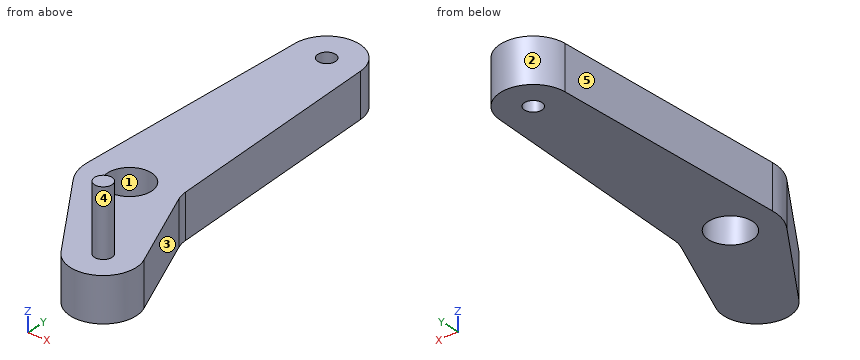
```python
from build123d import *

# Parameters (mm, degrees)
SKETCH_1_R      = 10
SKETCH_1_R_2    = 4
EXTRUDE_1_DEPTH = 20
SKETCH_2_R      = 4
EXTRUDE_2_DEPTH = 30


with BuildPart() as part:
    # 草图1 → 凸台-拉伸1 (new body)
    with BuildSketch(Plane.XY):
        with BuildLine():
            Line((-14.98449612, 110.681818182), (-19.97932816, 0.909090909))
            ThreePointArc((-19.97932816, 0.909090909), (-19.236072743, -5.474806428), (-16.506376679, -11.293340025))
            Line((-16.506376679, -11.293340025), (11.58545194, -52.352433595))
            ThreePointArc((11.58545194, -52.352433595), (31.154804784, -57.04715715), (37.782931026, -38.045369273))
            Line((37.782931026, -38.045369273), (20.861374384, 2.011947794))
            ThreePointArc((20.861374384, 2.011947794), (20.049111843, 4.537769231), (19.694574841, 7.167188916))
            Line((19.694574841, 7.167188916), (14.98449612, 110.681818182))
            ThreePointArc((14.98449612, 110.681818182), (0, 125), (-14.98449612, 110.681818182))
        make_face()
        Circle(SKETCH_1_R, mode=Mode.SUBTRACT)
        with Locations((0, 110)):
            Circle(SKETCH_1_R_2, mode=Mode.SUBTRACT)
    extrude(amount=EXTRUDE_1_DEPTH)

    # 草图2 → 凸台-拉伸2 (add)
    with BuildSketch(Plane.XY.offset(20)):
        with Locations((23.965234449, -43.882428577)):
            Circle(SKETCH_2_R)
    extrude(amount=EXTRUDE_2_DEPTH)


solid = part.part
```
Input: part model. Units: mm. Frame: model coordinates. Face numbers are marked on the shaded views. A direction names the side the tool comes from. Give positions to 0.01 mm unless a question says otherwise; leave off trailing zeros. Loops run counter-clockwise (first coordinate to the right, second up) from the corner with the lowest first, then second, coordinate; pieces in that order, holes last. Notation, with made-up numbers: M 24,-10.5 L 35,-10.5 A30 cw 35,16.5 Z; hole C -33,19.5 d6. An arc over 180 degrees is marked long. Answer as CSV lines item,"result". Start each with the question number.
1. Section B-B on z = 12. Return loops of the section in (x, y).
2. Line query: L1, parallel to Y at x = 24, z = 27; L2, parallel to Z at x = 2, y = -36; L3, parallel to Y at x = 33.5, z = 5. Output: solid intervals per line, ascending.
3. Pin query (flat end, axial travel): P1, Ø1.5, axis at y = 12.5, z = 17, coming from the -X side; P2, Ø10, axis at x = -2, z = 20, coming from the -Y side; P3, Ø8, axis at x = 26.5, z = 45, coming from the +Y side. Return the tip coordinate at first contact, or that it passes through.
4. Pull-direction query (X, two-part tool) for the marked faces 1, 2 and 3; classes: released by +X, released by -X, zero draft, split by the parting line, or undercut.
5. Reachability of the marked faces 4 and 5 from +Z, -Z, +X, -X, +Y, -Y: full face, straight path, thin tool, end or side. Return the list, or none.
6. Section C-C on y = 104. Return loops of the section in (x, z).
7. Section A-A on x = 0. Return loops of the section in (y, z), plus the area to 3 significant figures.
8. Section D-D on x = 35. Return loops of the section in (y, z), plus the area to 3 significant figures.
Computed values:
1,outline,"M -19.98,0.91 A20 ccw -16.51,-11.29 L 11.59,-52.35 A15 ccw 37.78,-38.05 L 20.86,2.01 A15 cw 19.69,7.17 L 14.98,110.68 A15 ccw -14.98,110.68 Z; hole C 0,0 d20; hole C 0,110 d8"
2,L1,"y = -47.88 to -39.88"
2,L2,"z = 0 to 20"
2,L3,"y = -55.46 to -27.91"
3,P1,"stops at x = -19.49"
3,P2,"stops at y = -39.8"
3,P3,"stops at y = -39.88"
4,face 1,"undercut"
4,face 2,"split by the parting line"
4,face 3,"released by +X"
5,face 4,"+Z"
5,face 5,"+Z, -Z, -X, +Y"
6,outline,"M -15.29,0 L 15.29,0 L 15.29,20 L -15.29,20 Z"
7,outline,"M -35.42,0 L -10,0 L -10,20 L -35.42,20 Z; M 10,0 L 106,0 L 106,20 L 10,20 Z; M 114,0 L 125,0 L 125,20 L 114,20 Z"
7,area,"2,650 mm²"
8,outline,"M -54.04,0 L -31.46,0 L -31.46,20 L -54.04,20 Z"
8,area,"452 mm²"
